from build123d import *

# Parameters (mm, degrees)
PAD021_DEPTH = 4
FILLET017_R  = 3


with BuildPart() as fillet017:
    # Sketch025 → Pad021 (new body)
    with BuildSketch(Plane.XZ.offset(15)):
        Polygon((-5.834702, 2.479193), (2.126768, 5.596979), (22.829249, -38.220491), (14.867778, -41.338277), align=None)
    extrude(amount=PAD021_DEPTH)

    # Fillet017
    fillet017_edges = [fillet017.edges().sort_by_distance(p)[0] for p in [
        (-5.834702, -17, 2.479193),
        (2.126768, -17, 5.596979),
        (22.829249, -17, -38.220491),
        (14.867778, -17, -41.338277),
    ]]
    fillet(fillet017_edges, radius=FILLET017_R)


with BuildPart() as part_mirroring013:
    # Part__Mirroring013: instance of Fillet017
    add(fillet017.part.mirror(Plane(origin=(0, 0, 0), x_dir=(0, -1, 0), z_dir=(1, 0, 0))))


with BuildPart() as part_mirroring013_1:
    # Part__Mirroring013 placement: moved
    add(part_mirroring013.part.moved(Location((76, 0, 0))))


solid = part_mirroring013_1.part
Geometry: final body of the model. Coordinates: model frame, mm. Coordinates: 2 decimals unless noted, no trailing zeros. Order: outer loops, then holes, each group sorted by start corner. A loop starts at its lowest first (then second) coordinate and runs counter-clockwise, first axis right, second up.
1) Section A-A (y = -17.9). Return loops of the section in (x, z), then the cut area to 3 significant figures.
Result sheet:
outline: (54.54, -35.32) arc R3 ccw to (56.16, -39.39) - (58.52, -40.32) arc R3 ccw to (62.33, -38.8) - (80.46, -0.42) arc R3 ccw to (78.84, 3.65) - (76.48, 4.58) arc R3 ccw to (72.68, 3.06) - close
area: 406 mm2
2) Section C-C (z = -29.5). Return loops of the section in (x, y), then the cut area to 3 significant figures.
Result sheet:
outline: (57.29, -19) - (66.73, -19) - (66.73, -15) - (57.29, -15) - close
area: 37.7 mm2
3) Draft query along X for faces 1 (the flat face through (67, -15, -18)), 2 (the flat face through (63.736, -16.972, -15.858)), 3 (the flat face through (77.7, -17, 4.1)). Return one class per face: released by +X, released by -X, zero draft, split by the parting line, or undercut.
Result sheet:
face 1: zero draft
face 2: released by -X
face 3: released by +X
4) Ray query, probe 1 along Z at (x, y) = (63, -16.2); probe 2 along Z at (x, y) = (69.75, -18.15); probe 3 along X at (y, z) = (-16.5, -22). Return the intervals inside material, ascending.
Result sheet:
probe 1: z = -37.39 to -17.42
probe 2: z = -23.1 to -3.13
probe 3: x = 60.83 to 70.27
5) Section B-B (x = 67). Return loops of the section in (y, z), then the cut area to 3 significant figures.
Result sheet:
outline: (-19, -28.92) - (-15, -28.92) - (-15, -8.95) - (-19, -8.95) - close
area: 79.9 mm2
6) First-contact query: P1, Ø2, axis at y = -17, z = -2.5, coming from the +X side; P2, Ø2, axis at y = -17, z = -32, coming from the -X side; P3, Ø1, axis at y = -17, z = -13.5, coming from the -X side. Flat tips, straight axial feed; report the tip coordinate or a pass-through.
Result sheet:
P1: stops at x = 79.95
P2: stops at x = 55.64
P3: stops at x = 64.61
